The model under review builds one solid part; all positions refer to its coordinate system, in mm. Round coordinates to 2 decimals unless told otherwise and drop trailing zeros. Write each loop counter-clockwise with the first axis right and the second up, starting at its lowest first coordinate (ties: lowest second). Pieces come first, ordered by that corner, then holes.
Item 1: Add section C-C (y = 5). Give the boundary of the cut face in (x, z) (3 decimals), plus the area to 3 significant figures.
Item 2: Draft analysis for pull direction Z (two halves, no side actions). For faces 1 (the face through (20, 5, -7.75)), 2 (the face through (38.85, 4.94, -3.11)), 3 (the face through (2.66, 4.94, -2.66)), 4 (the face through (20, 0, -4)), state which applies: +Z half, -Z half, draft (parallel to the pull), parting line (faces both ways), or undercut.
Item 3: Add section B-B (z = -3.5). Give the boundary of the cut face in (x, y), plus the area to 3 significant figures.
Item 4: Add section A-A (x = 4.25). Give the boundary of the cut face in (y, z) (3 decimals).
Item 5: To check wall thickness, follow L1, parallel to Z at x = 4.25, y = 6.25 (3 decimals); L2, parallel to X at y = 8.75, z = -3.5; L3, parallel to X at y = 4, z = -3.25. State the ranges of each line that lie inside material, in increasing order.
```python
from build123d import *

# Parameters (mm, degrees)
SKETCH1_W           = 7.75
SKETCH1_H           = 9.75
BOSS_EXTRUDE1_DEPTH = 40
SKETCH4_R           = 2
CUT_EXTRUDE3_DEPTH  = 9.75
CHAMFER1_SIZE       = 0.5


with BuildPart() as part:
    # Sketch1 → Boss-Extrude1 (new body)
    with BuildSketch(Plane(origin=(0, 0, 0), x_dir=(0, 0, -1), z_dir=(1, 0, 0))):
        with Locations((3.875, 4.875)):
            Rectangle(SKETCH1_W, SKETCH1_H)
    extrude(amount=BOSS_EXTRUDE1_DEPTH)

    # Sketch4 → Cut-Extrude3 (cut)
    with BuildSketch(Plane(origin=(0, 9.75, 0), x_dir=(1, 0, 0), z_dir=(0, 1, 0))):
        with Locations((4.25, 3.875)):
            Circle(SKETCH4_R)
        with Locations((37, 3.875)):
            Circle(SKETCH4_R)
    extrude(amount=-CUT_EXTRUDE3_DEPTH, mode=Mode.SUBTRACT)

    # Chamfer1
    chamfer1_edges = [part.edges().sort_by_distance(p)[0] for p in [
        (40, 4.875, -7.75),
        (40, 9.75, -3.875),
        (40, 4.875, 0),
        (0, 9.75, -3.875),
        (0, 4.875, -7.75),
        (0, 0, -3.875),
        (0, 4.875, 0),
        (20, 9.75, 0),
        (20, 9.75, -7.75),
        (20, 0, -7.75),
        (20, 0, 0),
        (40, 0, -3.875),
    ]]
    chamfer(chamfer1_edges, length=CHAMFER1_SIZE)


solid = part.part
```
Numbers:
1. outline: (0, -7.25) - (0.5, -7.75) - (39.5, -7.75) - (40, -7.25) - (40, -0.5) - (39.5, 0) - (0.5, 0) - (0, -0.5) - close; hole circle Ø4 at (4.25, -3.875); hole circle Ø4 at (37, -3.875)
1. area: 284 mm2
2. face 1: -Z half
2. face 2: undercut
2. face 3: undercut
2. face 4: draft
3. outline: (0, 0.5) - (0.5, 0) - (2.29, 0) - (2.29, 9.75) - (0.5, 9.75) - (0, 9.25) - close; (6.21, 0) - (35.04, 0) - (35.04, 9.75) - (6.21, 9.75) - close; (38.96, 0) - (39.5, 0) - (40, 0.5) - (40, 9.25) - (39.5, 9.75) - (38.96, 9.75) - close
3. area: 313 mm2
4. outline: (0, -7.25) - (0.5, -7.75) - (9.25, -7.75) - (9.75, -7.25) - (9.75, -5.875) - (0, -5.875) - close; (0, -1.875) - (9.75, -1.875) - (9.75, -0.5) - (9.25, 0) - (0.5, 0) - (0, -0.5) - close
5. L1: z = -7.75 to -5.875, -1.875 to 0
5. L2: x = 0 to 2.29, 6.21 to 35.04, 38.96 to 40
5. L3: x = 0 to 2.35, 6.15 to 35.1, 38.9 to 40
